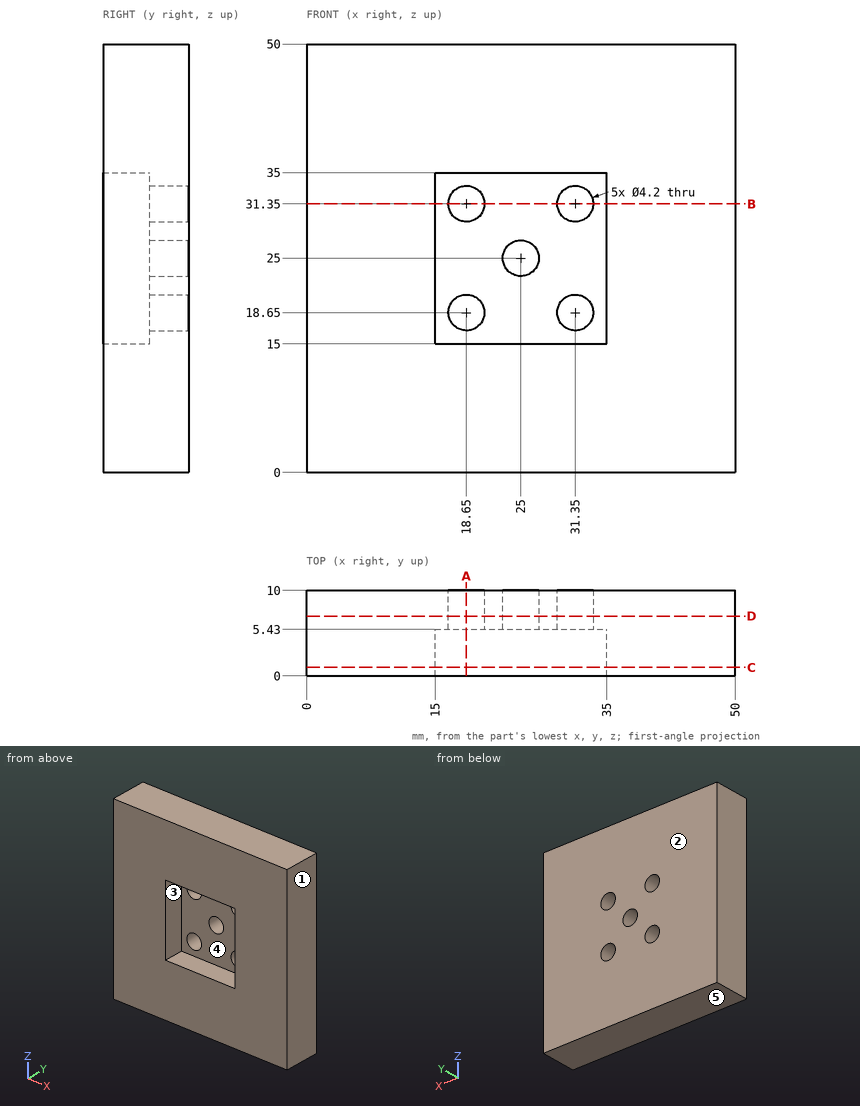
Verification items for this drawing (mm, ordinates from the low corner). A direction names the side the tool comes from. Coordinates: 2 decimals unless noted, no trailing zeros. Order: outer loops, then holes, each group sorted by start corner. A loop starts at its lowest first (then second) coordinate and runs counter-clockwise, first axis right, second up. Notation, with made-up numbers: M 32.25,25.25 L 48.25,25.25 A12 cw 48.25,35.25 Z; hole C 10.25,12 d3. An arc over 180 degrees is marked long. One line per item, written item: value. Start each with the question number.
Item 1: Thickness scan on probe 1 along X at (y, z) = (7, 31.35); probe 2 along X at (y, z) = (8.05, 25). Record the ranges inside material, lowest first.
Item 2: Mould release check, pull along X, two halves, no side actions. Record for the marked faces 1, 2 and 3: pulls with the +X half, pulls with the -X half, needs draft (parallel to the pull), parting line crosses it, or undercut.
Item 3: Depth check by flat-ended pin: P1, Ø2.5, axis at x = 18.65, z = 31.35, coming from the -Y side; P2, Ø10, axis at x = 27, z = 23.5, coming from the -Y side. Enter the tip coordinate at first touch or a pass-through.
Item 4: Sectioned sample at A-A on x = 18.65. Record the cut outline in (y, z), then the cut area to 3 significant figures.
Item 5: Access from +Z, -Z, +X, -X, +Y, -Y to the whole of each face (thin tool, end or side, straight path). Record for the marked faces 4 and 5.
Item 6: Sectioned sample at B-B on z = 31.35. Record the cut outline in (x, y), then the cut area to 3 significant figures.
Item 7: Sectioned sample at D-D on y = 7. Record the cut outline in (x, z), then the cut area to 3 significant figures.
Item 8: Sectioned sample at C-C on y = 1. Record the cut outline in (x, z), then the cut area to 3 significant figures.
Calculated:
1. probe 1: 0 to 16.55, 20.75 to 29.25, 33.45 to 50
1. probe 2: 0 to 22.9, 27.1 to 50
2. face 1: pulls with the +X half
2. face 2: needs draft
2. face 3: undercut
3. P1: through
3. P2: y = 5.43
4. outline: M 0,0 L 10,0 L 10,16.55 L 5.43,16.55 L 5.43,15 L 0,15 Z; M 0,35 L 5.43,35 L 5.43,33.45 L 10,33.45 L 10,50 L 0,50 Z; M 5.43,20.75 L 10,20.75 L 10,29.25 L 5.43,29.25 Z
4. area: 353 mm^2
5. face 4: -Y
5. face 5: -Z, +X, -X, +Y, -Y
6. outline: M 0,0 L 15,0 L 15,5.43 L 16.55,5.43 L 16.55,10 L 0,10 Z; M 20.75,5.43 L 29.25,5.43 L 29.25,10 L 20.75,10 Z; M 33.45,5.43 L 35,5.43 L 35,0 L 50,0 L 50,10 L 33.45,10 Z
6. area: 353 mm^2
7. outline: M 0,0 L 50,0 L 50,50 L 0,50 Z; hole C 18.65,18.65 d4.2; hole C 18.65,31.35 d4.2; hole C 25,25 d4.2; hole C 31.35,18.65 d4.2; hole C 31.35,31.35 d4.2
7. area: 2,430 mm^2
8. outline: M 0,0 L 50,0 L 50,50 L 0,50 Z; hole M 15,15 L 35,15 L 35,35 L 15,35 Z
8. area: 2,100 mm^2
